```python
from build123d import *

# Parameters (mm, degrees)
SALIENTE_EXTRUIR1_DEPTH = 5
CROQUIS2_R              = 2.1
CORTAR_EXTRUIR1_DEPTH   = 2.2
CROQUIS3_R              = 1
CORTAR_EXTRUIR2_DEPTH   = 10


with BuildPart() as part:
    # Croquis1 → Saliente-Extruir1 (new body)
    with BuildSketch(Plane(origin=(0, 0, 0), x_dir=(1, 0, 0), z_dir=(0, 1, 0))):
        with BuildLine():
            Line((-10, 0), (10, 0))
            Line((10, 0), (10, 10))
            Line((10, 10), (25.36, 10))
            ThreePointArc((25.36, 10), (0, 35.36), (-25.36, 10))
            Line((-25.36, 10), (-10, 10))
            Line((-10, 10), (-10, 0))
        make_face()
    extrude(amount=SALIENTE_EXTRUIR1_DEPTH)

    # Croquis2 → Cortar-Extruir1 (cut)
    with BuildSketch(Plane(origin=(0, 5, 0), x_dir=(1, 0, 0), z_dir=(0, 1, 0))):
        with Locations(Location((0, 30.2, 0), (0, 0, 270))):
            Circle(CROQUIS2_R)
        with Locations(Location((8.66, 15.2, 0), (0, 0, 270))):
            Circle(CROQUIS2_R)
        with Locations(Location((-8.66, 15.2, 0), (0, 0, 270))):
            Circle(CROQUIS2_R)
    extrude(amount=-CORTAR_EXTRUIR1_DEPTH, mode=Mode.SUBTRACT)

    # Croquis3 → Cortar-Extruir2 (cut)
    with BuildSketch(Plane(origin=(0, 5, 0), x_dir=(1, 0, 0), z_dir=(0, 1, 0))):
        with Locations(Location((-8.66, 15.2, 0), (0, 0, 270))):
            Circle(CROQUIS3_R)
        with Locations(Location((8.66, 15.2, 0), (0, 0, 270))):
            Circle(CROQUIS3_R)
        with Locations(Location((0, 30.2, 0), (0, 0, 270))):
            Circle(CROQUIS3_R)
    extrude(amount=-CORTAR_EXTRUIR2_DEPTH, mode=Mode.SUBTRACT)


solid = part.part
```
Could you check a few things on this model? Use its own coordinates, in mm. A direction names the side the tool comes from. Coordinates: 2 decimals unless noted, no trailing zeros. Loops run counter-clockwise (first coordinate to the right, second up) from the corner with the lowest first, then second, coordinate; pieces in that order, holes last.
1) Imagine slicing it at C-C (z = -3). List the corners of the cut face in (x, y) for me, and give its area (3 significant figures).
Reported:
outline: (-10, 0) - (10, 0) - (10, 5) - (-10, 5) - close
area: 100 mm2
2) Imagine slicing it at A-A (y = 1.9). List the corners of the cut face in (x, z) for me.
Reported:
outline: (-25.36, -10) arc R25.36 ccw to (25.36, -10) - (10, -10) - (10, 0) - (-10, 0) - (-10, -10) - close; hole circle Ø2 at (-8.66, -15.2); hole circle Ø2 at (0, -30.2); hole circle Ø2 at (8.66, -15.2)
3) Which directions (+Z, -Z, +X, -X, +Y, -Y) give clear straight access to the entire face, cutting with the end or side of a thin tool? Please do faces 1 (the face through (-9.938, 3.915, -16.866)), 2 (the face through (-10, 2, -5)), 3 (the face through (18, 2, -10)).
Reported:
face 1: +Y
face 2: +Z, -X, +Y, -Y
face 3: +Z, +X, +Y, -Y
4) Imagine slicing it at B-B (x = 0). List the corners of the cut face in (y, z) for me, and give its area (3 significant figures).
Reported:
outline: (0, -35.36) - (5, -35.36) - (5, -32.3) - (2.8, -32.3) - (2.8, -31.2) - (0, -31.2) - close; (0, -29.2) - (2.8, -29.2) - (2.8, -28.1) - (5, -28.1) - (5, 0) - (0, 0) - close
area: 162 mm2
5) Will these pins go through, and if not, where does the flat tip stop? pin 1 Ø1.8 at (x, z) = (0, -30.2) entering from -Y; pin 2 Ø3 at (x, z) = (8.66, -15.2) entering from +Y; pin 3 Ø2 at (y, z) = (1, -3.5) entering from -X; pin 4 Ø2.5 at (x, y) = (-21, 2) entering from +Z.
Reported:
pin 1: passes through
pin 2: stops at y = 2.8
pin 3: stops at x = -10
pin 4: stops at z = -10
6) Please list where these lines run through material, in increasing order: line 1 along X through (y, z) = (4.3, -15.2); line 2 along X through (y, z) = (2, -15.2); line 3 along X through (y, z) = (0.6, -2).
Reported:
line 1: x = -24.82 to -10.76, -6.56 to 6.56, 10.76 to 24.82
line 2: x = -24.82 to -9.66, -7.66 to 7.66, 9.66 to 24.82
line 3: x = -10 to 10
7) Thinking about a two-plate mould opening in X: for faces 4 (the face through (10, 2, -5)), 5 (the face through (0.558, 2.465, -35.354)), 6 (the face through (-18, 2, -10)), 7 (the face through (7.77, 1.42, -14.74)), which applies, released by +X, released by -X, zero draft, split by the parting line, or undercut?
Reported:
face 4: released by +X
face 5: split by the parting line
face 6: zero draft
face 7: undercut
8) Imagine slicing it at D-D (x = 8.66). List the corners of the cut face in (y, z) for me, and give its area (3 significant figures).
Reported:
outline: (0, -33.84) - (5, -33.84) - (5, -17.3) - (2.8, -17.3) - (2.8, -16.2) - (0, -16.2) - close; (0, -14.2) - (2.8, -14.2) - (2.8, -13.1) - (5, -13.1) - (5, 0) - (0, 0) - close
area: 154 mm2
